Autodesk Inventor part; units mm, degrees
ref_plane "YZ Plane" through (0, 0, 0) normal (1, 0, 0) x (0, 1, 0)
ref_plane "XZ Plane" through (0, 0, 0) normal (0, 1, 0) x (-1, 0, 0)
ref_plane "XY Plane" through (0, 0, 0) normal (0, 0, 1) x (1, 0, 0)
sketch "草圖5" plane through (0, 0, 0) normal (0, 0, 1) x (1, 0, 0)
  line L0 (0, 14.1091) -> (0, -11.8545)
  line L1 (-92, 0) -> (-102, 0)
  line L2 (-102, 0) -> (-108.9282, 4)
  line L3 (-108.9282, 4) -> (-116, 4)
  line L4 (-116, 4) -> (-116, 6)
  line L5 (-116, 6) -> (-108.3923, 6)
  line L6 (-108.3923, 6) -> (-101.4641, 2)
  line L7 (-101.4641, 2) -> (-92, 2)
  line L8 (-92, 4.8545) -> (-92, -2.1478) construction
  line L9 (-92, 0) -> (-82, 0)
  line L10 (-82, 0) -> (-82, 2)
  line L11 (-82, 2) -> (-92, 2)
  point P0 (0, 0)
  point P1 (0, 2)
  dimension "d26" = 2
  dimension "d27" = 232
  dimension "d28" = 92
  dimension "d31" = 2
  dimension "d32" = 2
  dimension "d33" = 4
  dimension "d34" = 30
  dimension "d35" = 20
revolve "迴轉1" add sketch "草圖5" angle 360 about axis through (0, 14.1091, 0) along (0, -1, 0)
sketch "草圖6" plane through (0, 0, 0) normal (0, 1, 0) x (-1, 0, 0)
  circle A0 centre (0, -92) radius 2.58
  line L0 (0, -136.9187) -> (0, 28.2306) construction
  line L1 (-16.0697, -114.8815) -> (-9.2729, -89.5153)
  arc A1 (7.341, -90.033) -> (-7.341, -90.033) centre (0, -92) ccw
  line L2 (16.0697, -114.8815) -> (9.2729, -89.5153)
  arc A2 (-16.0697, -114.8815) -> (16.0697, -114.8815) centre (0, 0) ccw
  circle A3 centre (0, 0) radius 116 construction
  arc A4 (9.2729, -89.5153) -> (-9.2729, -89.5153) centre (0, -92) ccw
  arc A5 (-9.7984, -91.4767) -> (9.7984, -91.4767) centre (0, 0) ccw construction
  line L3 (-7.341, -90.033) -> (-9.2729, -89.5153)
  line L4 (7.341, -90.033) -> (9.2729, -89.5153)
  arc A6 (7.2444, -90.0589) -> (-7.2207, -89.9724) centre (0, -92) ccw construction
  point P0 (-9.2729, -89.5153)
  dimension "d38" = 92
  dimension "d46" = 5.16
  dimension "d81" = 7.6
  dimension "d82" = 2
  dimension "d83" = 30
  dimension "d88" = 7.5
extrude "擠出5" cut sketch "草圖6" along normal up to next contours A0
extrude "擠出8" cut sketch "草圖6" along normal blind 10 keep common part
extrude "擠出9" add sketch "草圖6" against normal blind 3 contours A4 L4 A1 L3
fillet "圓角5" radius 2 2 edges at (8.307, 0, -89.7742) (-8.307, 0, -89.7742)
properties part number "transmission_support"
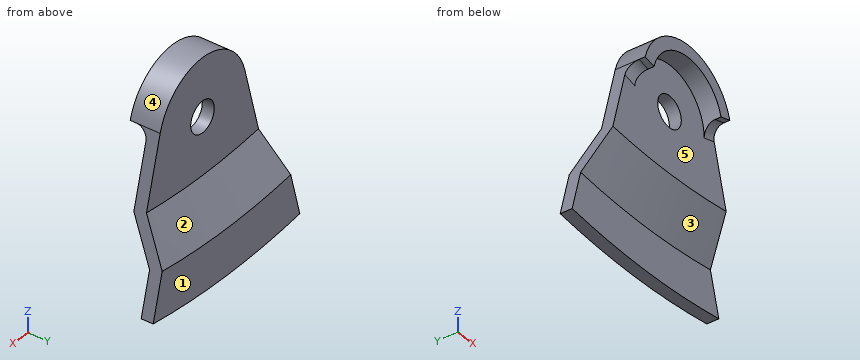
Design review of the part built by this model. Coordinates are the model's own, in mm. Face numbers are marked on the shaded views. A direction names the side the tool comes from. Give positions to 0.01 mm unless a question says otherwise; leave off trailing zeros. Order: outer loops, then holes, each group sorted by start corner. A loop starts at its lowest first (then second) coordinate and runs counter-clockwise, first axis right, second up. Notation, with made-up numbers: (31.25, 89) - (58.25, 89) arc R18 cw to (58.25, 101) - close; hole circle Ø1 at (89, 45.25). An arc over 180 degrees is marked (long way). Use a Markdown table: item, result. Add a question column.
(1) Machinability: for the marked faces 4 and 5, which of the approach directions +Z, -Z, +X, -X, +Y, -Y give a long, thin tool a straight path to every point of the face, cutting with its end or side? Answer none if there is none.
(2) Clearance check with flat-ended pins moving along their axes: P1, Ø9, axis at x = 4, z = -93.5, coming from the -Y side; P2, Ø4, axis at x = 6, z = -112.5, coming from the -Y side; P3, Ø2, axis at x = -9.5, z = -95.5, coming from the -Y side; P4, Ø3, axis at x = 0, z = -92, coming from the -Y side. State where each tip first meets the part, or that it passes through.
(3) Add section A-A on x = 0. Give the boundary of the cut face in (y, z).
(4) Add section D-D on y = -0.75. Give the boundary of the cut face in (x, z), then the cut area to 3 significant figures.
(5) Wall thickness on probe 1 along Y at (x, z) = (2, -113.5); probe 2 along Y at (x, z) = (4, -97); probe 3 along Z at (x, y) = (0, 0.5): over which ranges is each line inside the solid? List them lowest first. Write a range as [from, to].
(6) Add section B-B on z = -85. Give the boundary of the cut face in (x, y).
(7) Mouldability with a two-part tool opening along X and no side actions: class the marked faces 1, 2 and 3 as +X half, -X half, draft (parallel to the pull), parting line (faces both ways), or undercut.
(8) Add section C-C on y = -2.5. Give the boundary of the cut face in (x, z).
Report:
| question | item | result |
|---|---|---|
| 1 | face 4 | +Z, +Y, -Y |
| 1 | face 5 | -Z, -Y |
| 2 | P1 | stops at y = -0.55 |
| 2 | P2 | stops at y = 4 |
| 2 | P3 | stops at y = 0 |
| 2 | P4 | passes through |
| 3 | outline | (-3, -84.4) - (0, -84.4) - (0, -89.42) - (2, -89.42) - (2, -82.4) - (-3, -82.4) - close; (0, -102) - (4, -108.93) - (4, -116) - (6, -116) - (6, -108.39) - (2, -101.46) - (2, -94.58) - (0, -94.58) - close |
| 4 | outline | (-9.39, -89.94) - (-7.44, -90.46) arc R7.6 cw to (7.44, -90.46) - (9.39, -89.94) - (9.27, -89.52) arc R9.6 ccw to (-9.27, -89.52) - close |
| 4 | area | 46.8 mm² |
| 5 | probe 1 | y = [4, 6] |
| 5 | probe 2 | y = [0, 2] |
| 5 | probe 3 | z = [-102.87, -94.58], [-89.42, -82.4] |
| 6 | outline | (-6.57, -3) - (-2.96, -3) - (-2.96, 0) - (2.96, 0) - (2.96, -3) - (6.57, -3) - (6.57, 2) - (-6.57, 2) - close |
| 7 | face 1 | draft |
| 7 | face 2 | undercut |
| 7 | face 3 | parting line |
| 8 | outline | (-9.27, -89.52) - (-7.34, -90.03) arc R7.6 cw to (7.34, -90.03) - (9.27, -89.52) arc R9.6 ccw to start |
